Could you check a few things on this model? Use its own coordinates, in mm. Face numbers are marked on the shaded views. A direction names the side the tool comes from. Coordinates: 2 decimals unless noted, no trailing zeros. Loops run counter-clockwise (first coordinate to the right, second up) from the corner with the lowest first, then second, coordinate; pieces in that order, holes last. Notation, with made-up numbers: M 64,79.25 L 79,79.25 A13 ccw 79,88.25 Z; hole C 54.25,21.5 d10. An arc over 180 degrees is marked long. Write each question's results on one line, items separated by ' | '.
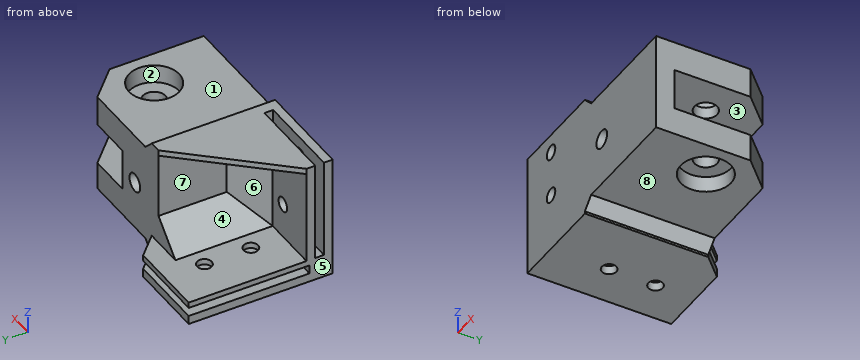
Autodesk Inventor part; units mm, degrees
ref_plane "Work Plane3" through (-127, -182.5, -3.81) normal (0, 0, -1) x (0, 1, 0)
ref_plane "YZ Plane" through (0, 0, 0) normal (1, 0, 0) x (0, 1, 0)
ref_plane "XZ Plane" through (0, 0, 0) normal (0, 1, 0) x (-1, 0, 0)
ref_plane "Work Plane1" through (0, 0, 0) normal (0, 0, 1) x (1, 0, 0)
ref_plane "Work Plane2" through (127, 182.5, 0) normal (1, 0, 0) x (0, 1, 0)
sketch "Sketch1" plane through (127, 182.5, 0) normal (1, 0, 0) x (0, 1, 0)
  line L0 (0, -3.81) -> (-365, -3.81)
  line L1 (0, 0) -> (0, -3.81)
  line L2 (0, 0) -> (-365, 0)
  line L3 (-365, 0) -> (-365, -3.81)
  line L4 (-371.35, 459.74) -> (-371.35, 2.54)
  line L5 (-367.54, 2.54) -> (-371.35, 2.54)
  line L6 (-367.54, 459.74) -> (-367.54, 2.54)
  line L7 (-367.54, 459.74) -> (-371.35, 459.74)
  line L8 (-367.54, 46.355) -> (-363.73, 46.355)
  line L9 (-321.185, -3.81) -> (-321.185, -7.62)
  line L10 (-321.185, -7.62) -> (-375.16, -7.62)
  line L11 (-375.16, -7.62) -> (-375.16, 46.355)
  line L12 (-363.73, 46.355) -> (-363.73, 2.54)
  line L13 (-363.73, 2.54) -> (-321.185, 2.54)
  line L14 (-321.185, 2.54) -> (-321.185, 0)
  line L15 (-321.185, 0) -> (-365, 0)
  line L16 (-365, 0) -> (-365, -3.81)
  line L17 (-365, -3.81) -> (-321.185, -3.81)
  line L18 (-371.35, 46.355) -> (-371.35, 41.275)
  line L19 (-371.35, 41.275) -> (-371.35, 2.54)
  line L20 (-371.35, 2.54) -> (-367.54, 2.54)
  line L21 (-367.54, 2.54) -> (-367.54, 46.355)
  line L22 (-375.16, 46.355) -> (-371.35, 46.355)
  line L23 (-367.54, 46.355) -> (-363.73, 46.355)
  point P0 (-182.5, 0)
  point P1 (-326.265, 0)
  point P2 (-326.265, -3.81)
  point P3 (-367.54, 41.275)
  dimension "d2" = 3.81
  dimension "d4" = 3.81
extrude "Extrusion1" add sketch "Sketch1" against normal blind 38.1 contours L9 L10 L11 L22 L4 L5 L6 L8 L12 L13 L14 L2 L3 L0
sketch "Sketch2" plane through (127, 182.5, 0) normal (1, 0, 0) x (0, 0, -1)
  line L0 (3.81, -365) -> (0, -365)
  line L1 (0, -365) -> (0, -321.185)
  line L2 (0, -321.185) -> (-2.54, -321.185)
  line L3 (-2.54, -321.185) -> (-2.54, -363.73)
  line L4 (-2.54, -363.73) -> (-46.355, -363.73)
  line L5 (-46.355, -363.73) -> (-46.355, -367.54)
  line L6 (-46.355, -367.54) -> (-2.54, -367.54)
  line L7 (-2.54, -367.54) -> (-2.54, -371.35)
  line L8 (-2.54, -371.35) -> (-46.355, -371.35)
  line L9 (-46.355, -371.35) -> (-46.355, -375.16)
  line L10 (-46.355, -375.16) -> (7.62, -375.16)
  line L11 (7.62, -375.16) -> (7.62, -321.185)
  line L12 (7.62, -321.185) -> (3.81, -321.185)
  line L13 (3.81, -321.185) -> (3.81, -365)
  line L14 (3.81, -321.185) -> (7.62, -321.185)
  line L15 (7.62, -375.16) -> (-46.355, -375.16)
  line L16 (7.62, -321.185) -> (-46.355, -321.185)
  line L17 (-46.355, -321.185) -> (-46.355, -375.16)
  line L18 (-46.355, -375.16) -> (7.62, -375.16)
  line L19 (7.62, -375.16) -> (7.62, -321.185)
  point P0 (0, -182.5)
extrude "Extrusion2" add sketch "Sketch2" along normal blind 5.08
sketch "Sketch3" plane through (88.9, -138.685, -3.81) normal (0, 1, 0) x (1, 0, 0)
  line L0 (38.1, -3.81) -> (0, -3.81)
  line L1 (0, -6.35) -> (0, -3.81)
  line L2 (38.1, -6.35) -> (0, -6.35)
  line L3 (38.1, -6.35) -> (38.1, -50.165)
  line L4 (38.1, -50.165) -> (43.18, -50.165)
  line L5 (43.18, 3.81) -> (43.18, -50.165)
  line L6 (0, 3.81) -> (43.18, 3.81)
  line L7 (0, 0) -> (0, 3.81)
  line L8 (38.1, 0) -> (0, 0)
  line L9 (38.1, 0) -> (38.1, -3.81)
  line L10 (43.18, -50.165) -> (43.18, 3.81)
  line L11 (43.18, -23.1775) -> (55.88, -23.1775)
  circle A0 centre (55.88, -23.1775) radius 4
  line L12 (55.88, -27.1775) -> (55.88, -32.2575)
  line L13 (55.88, -19.1775) -> (55.88, -14.0975)
  line L14 (59.88, -23.1775) -> (64.96, -23.1775)
  line L15 (43.18, -14.0975) -> (64.96, -14.0975)
  line L16 (64.96, -14.0975) -> (64.96, -32.2575)
  line L17 (64.96, -32.2575) -> (43.18, -32.2575)
  line L18 (43.18, -32.2575) -> (43.18, -14.0975)
  point P0 (-88.9, -3.81)
  dimension "d9" = 12.7
  dimension "d10" = 8
  dimension "d11" = 5.08
  dimension "d12" = 5.08
  dimension "d13" = 5.08
extrude "Extrusion3" add sketch "Sketch3" against normal up to surface (53.975 mm away) contours L15 L13 A0 L11 L5 | L5 L11 A0 L12 L17 | L15 L16 L14 A0 L13 | L12 A0 L14 L16 L17
sketch "Sketch4" plane through (132.08, -138.685, 28.4475) normal (0, 0, 1) x (1, 0, 0)
  line L0 (0, -53.975) -> (21.78, -53.975)
  line L1 (21.78, 0) -> (21.78, -53.975)
  line L2 (0, 0) -> (21.78, 0)
  line L3 (0, -53.975) -> (0, 0)
  line L4 (0, -53.975) -> (0, 0)
  line L5 (21.78, 0) -> (21.78, -53.975)
  line L6 (0, -45.966) -> (21.78, -45.966)
  line L7 (21.78, -45.966) -> (21.78, -26.916)
  line L8 (21.78, -26.916) -> (0, -26.916)
  line L9 (0, -26.916) -> (0, -45.966)
  line L10 (21.78, -45.966) -> (53.53, -45.966)
  line L11 (53.53, -45.966) -> (53.53, 0)
  line L12 (53.53, 0) -> (21.78, 0)
  line L13 (21.78, 0) -> (21.78, -45.966)
  circle A0 centre (37.655, -22.983) radius 11
  point P0 (-132.08, 138.685)
  dimension "d16" = 19.05
  dimension "d17" = 31.75
  dimension "d18" = 22
extrude "Extrusion4" add sketch "Sketch4" along normal blind 5.08 contours L3 L8 L1 L6 | L1 L12 L11 L10 | L3 L2 L1 L8
sketch "Sketch5" plane through (153.86, -138.685, 10.2875) normal (0, 0, -1) x (-1, 0, 0)
  circle A0 centre (-15.875, -22.983) radius 11
  line L0 (21.78, -45.966) -> (-31.75, -45.966)
  line L1 (-31.75, -45.966) -> (-31.75, 0)
  line L2 (-31.75, 0) -> (21.78, 0)
  line L3 (21.78, -45.966) -> (21.78, 0)
  point P0 (153.86, 138.685)
extrude "Extrusion5" add sketch "Sketch5" along normal blind 5.08
sketch "Sketch6" plane through (132.08, -138.685, 33.5275) normal (0, 0, 1) x (1, 0, 0)
  circle A0 centre (37.655, -22.983) radius 11
  line L0 (0, -45.966) -> (53.53, -45.966)
  line L1 (53.53, -45.966) -> (53.53, 0)
  line L2 (53.53, 0) -> (0, 0)
  line L3 (0, -45.966) -> (0, 0)
  point P0 (-132.08, 138.685)
extrude "Extrusion6" add sketch "Sketch6" along normal blind 8
sketch "Sketch7" plane through (132.08, -138.685, 28.4475) normal (0, 0, -1) x (-1, 0, 0)
  line L0 (-53.53, -45.966) -> (-53.53, 0)
  circle A0 centre (-37.655, -22.983) radius 11
  line L1 (0, -45.966) -> (-53.53, -45.966)
  line L2 (-53.53, -45.966) -> (-53.53, 0)
  line L3 (-53.53, 0) -> (0, 0)
  line L4 (0, -45.966) -> (0, 0)
  circle A1 centre (-37.655, -22.983) radius 5
  point P0 (132.08, 138.685)
  dimension "d25" = 10
extrude "Extrusion7" add sketch "Sketch7" against normal blind 5.08 contours A0
chamfer "Chamfer1" distance 4.7625 angle 45 1 edges at (132.08, -161.668, 41.5275)
sketch "Sketch8" plane through (153.86, -138.685, 10.2875) normal (0, 0, 1) x (1, 0, 0)
  circle A0 centre (15.875, -22.983) radius 5
  circle A1 centre (15.875, -22.983) radius 11
  point P0 (-153.86, 138.685)
extrude "Extrusion8" add sketch "Sketch8" against normal blind 5.08
sketch "Sketch9" plane through (153.86, -138.685, 5.2075) normal (0, 0, -1) x (-1, 0, 0)
  circle A0 centre (-15.875, -22.983) radius 5
  line L0 (-31.75, -45.966) -> (21.78, -45.966)
  line L1 (21.78, 0) -> (21.78, -45.966)
  line L2 (21.78, 0) -> (-31.75, 0)
  line L3 (-31.75, 0) -> (-31.75, -45.966)
  circle A1 centre (-15.875, -22.983) radius 11
  point P0 (153.86, 138.685)
extrude "Extrusion9" add sketch "Sketch9" along normal blind 7 contours L3 L2 L1 L0
chamfer "Chamfer2" distance 4.7625 angle 45 1 edges at (132.08, -161.668, -1.7925)
sketch "Sketch10" plane through (153.86, -184.651, 28.4475) normal (0, -1, 0) x (1, 0, 0)
  line L0 (4.875, -23.24) -> (26.875, -23.24)
  line L1 (-21.78, -18.16) -> (0, -18.16)
  line L2 (-21.78, -35.0025) -> (-21.78, -18.16)
  line L3 (-17.0175, -30.24) -> (-21.78, -35.0025)
  line L4 (31.75, -30.24) -> (-17.0175, -30.24)
  line L5 (31.75, -18.16) -> (31.75, -30.24)
  line L6 (0, -18.16) -> (31.75, -18.16)
  line L7 (4.875, 5.08) -> (26.875, 5.08)
  line L8 (0, 0) -> (-21.78, 0)
  line L9 (0, 0) -> (31.75, 0)
  line L10 (31.75, 0) -> (31.75, 13.08)
  line L11 (-17.0175, 13.08) -> (31.75, 13.08)
  line L12 (-21.78, 17.8425) -> (-17.0175, 13.08)
  line L13 (-21.78, 0) -> (-21.78, 17.8425)
  line L14 (0, 0) -> (31.75, 0)
  line L15 (31.75, -30.24) -> (0, -30.24)
  line L16 (0, -30.24) -> (0, 0)
  line L17 (0, 0) -> (31.75, 0)
  line L18 (31.75, 0) -> (31.75, -30.24)
  point P0 (-153.86, -28.4475)
extrude "Extrusion10" add sketch "Sketch10" along normal up to surface (8.009 mm away)
sketch "Sketch11" plane through (88.9, -185.04, 46.355) normal (0, 0, 1) x (1, 0, 0)
  line L0 (38.1, 3.81) -> (0, 3.81)
  line L1 (0, 0) -> (0, 3.81)
  line L2 (38.1, 0) -> (0, 0)
  line L3 (38.1, 0) -> (38.1, -3.81)
  line L4 (38.1, -3.81) -> (0, -3.81)
  line L5 (0, -7.62) -> (0, -3.81)
  line L6 (0, -7.62) -> (43.18, -7.62)
  line L7 (43.18, 46.355) -> (43.18, -7.62)
  line L8 (38.1, 46.355) -> (43.18, 46.355)
  line L9 (38.1, 46.355) -> (38.1, 3.81)
  line L10 (0, 0) -> (0, 3.81)
  line L11 (38.1, 46.355) -> (0, 3.81)
  line L12 (38.1, 3.81) -> (0, 3.81)
  line L13 (0, 3.81) -> (38.1, 3.81)
  line L14 (38.1, 3.81) -> (38.1, 46.355)
  point P0 (-88.9, 185.04)
extrude "Extrusion11" add sketch "Sketch11" against normal blind 2.54 contours L0 L11 L9
sketch "Sketch12" plane through (88.9, -181.23, 2.54) normal (0, 0, 1) x (1, 0, 0)
  circle A0 centre (17.78, 13.97) radius 3.175
  circle A1 centre (17.78, 34.29) radius 3.175
  circle A2 centre (17.78, 13.97) radius 3.175
  point P0 (-88.9, 181.23)
extrude "Extrusion12" cut sketch "Sketch12" against normal blind 45.4025
sketch "Sketch13" plane through (88.9, -181.23, 2.54) normal (0, 1, 0) x (1, 0, 0)
  circle A0 centre (17.78, -15.24) radius 3.175
  circle A1 centre (17.78, -35.56) radius 3.175
  point P0 (-88.9, 2.54)
extrude "Extrusion13" cut sketch "Sketch13" along normal mid plane 45.4025
chamfer "Chamfer3" distance 12.7 angle 45 2 edges at (127, -159.9575, 2.54) (127, -181.23, 23.1775)
chamfer "Chamfer4" distance 12.7 angle 45 2 edges at (185.61, -138.685, 4.2475) (185.61, -138.685, 34.9875)
sketch "Sketch14" plane through (88.9, -192.66, -7.62) normal (0, 0, -1) x (-1, 0, 0)
  circle A0 centre (-17.78, 25.4) radius 3.175
  circle A1 centre (-17.78, 45.72) radius 3.175
  line L0 (0, 0) -> (-43.18, 0)
  line L1 (0, 53.975) -> (0, 0)
  line L2 (0, 53.975) -> (-43.18, 53.975)
  line L3 (-43.18, 0) -> (-43.18, 53.975)
  line L4 (-43.18, 53.975) -> (-34.1997, 62.9553)
  line L5 (-43.18, 53.975) -> (-30.48, 53.975) construction
  line L6 (-34.1997, 62.9553) -> (0, 62.9553)
  line L7 (-25.4, 53.975) -> (0, 53.975)
  line L8 (0, 62.9553) -> (0, 53.975)
  line L9 (-47.9425, 53.975) -> (-43.18, 53.975)
  line L10 (-43.18, 53.975) -> (0, 53.975)
  point P0 (88.9, 192.66)
  dimension "d52" = 12.7
  dimension "d53" = 45
ref_plane "Work Plane3" through (-127, -182.5, -3.81) normal (0, 0, -1) x (0, 1, 0)
extrude "Extrusion14" add sketch "Sketch14" against normal up to surface (3.81 mm away) contours L2 L4 L6 L8
sketch "Sketch15" plane through (88.9, -182.5, 0) normal (0, 0, -1) x (-1, 0, 0)
  line L0 (-43.18, 43.815) -> (-34.1997, 52.7953)
  line L1 (-34.1997, 52.7953) -> (0, 52.7953)
  line L2 (-25.4, 43.815) -> (0, 43.815)
  line L3 (-38.1, 43.815) -> (-25.4, 43.815)
  line L4 (-38.1, 43.815) -> (-43.18, 43.815)
  line L5 (0, 0) -> (0, 52.7953)
  point P0 (88.9, 182.5)
extrude "Extrusion15" add sketch "Sketch15" against normal up to surface (2.54 mm away)
properties part number "Ystartnew"
(1) Which directions (+Z, -Z, +X, -X, +Y, -Y) give clear straight access to the entire face, cutting with the end or side of a thin tool? Please do the marked faces 1, 2, 3 and 4.
Reported:
face 1: +Z, +X, +Y, -Y | face 2: +Z | face 3: +X, +Y | face 4: -X, +Y
(2) Will these pins go through, and if not, where does the flat tip stop? P1, Ø5, axis at x = 106.68, z = 38.1, coming from the +Y side; P2, Ø12, axis at x = 139.5, y = -142, coming from the -Z side (3 decimals); P3, Ø3, axis at x = 138.5, y = -172, coming from the +Z side; P4, Ø20.5, axis at x = 97, z = 32.5, coming from the +Y side.
Reported:
P1: passes through | P2: stops at z = -5.135 | P3: stops at z = 41.53 | P4: stops at y = -181.23
(3) Please list where these lines run through material, in increasing order: probe 1 along Z at (x, y) = (100, -131.5); probe 2 along Y at (x, z) = (99, 4); probe 3 along Y at (x, z) = (125.5, 5) (3 decimals). Write a range as from..to.
Reported:
probe 1: z = -7.62..-3.81, 0..2.54 | probe 2: y = -192.66..-188.85, -185.04..-181.23 | probe 3: y = -192.66..-188.85, -185.04..-138.685
(4) Imagine slicing it at C-C, the plane y = -146.94. State how many separate pieces and enclosed holes the cut face has, and give its area (3 significant figures).
Reported:
separate pieces: 3 | enclosed holes: 1 | area: 2,180 mm2
(5) Imagine slicing it at A-A, the plane x = 144.78. List the corners of the cut face in (y, z) for me (1 decimal).
Reported:
outline: M -192.7,-1.8 L -138.7,-1.8 L -138.7,15.4 L -192.7,15.4 Z; M -192.7,23.4 L -138.7,23.4 L -138.7,41.5 L -192.7,41.5 Z
(6) Imagine slicing it at B-B, the plane z = 38.1. List the corners of the cut face in (x, y) for me (3 decimals).
Reported:
outline: M 88.9,-192.66 L 103.505,-192.66 L 103.505,-188.85 L 88.9,-188.85 Z; M 88.9,-185.04 L 103.505,-185.04 L 103.505,-181.23 L 88.9,-181.23 Z; M 109.855,-192.66 L 185.61,-192.66 L 185.61,-151.385 L 172.91,-138.685 L 127,-138.685 L 127,-168.53 L 114.3,-181.23 L 109.855,-181.23 L 109.855,-185.04 L 127,-185.04 L 127,-188.85 L 109.855,-188.85 Z; hole C 169.735,-161.668 d22
(7) If we mould it in two halves opening along Z, with no side actions, what happens to the marked faces 5, 6, 7 and 8? For each: released by +Z, released by -Z, zero draft, split by the parting line, or undercut.
Reported:
face 5: zero draft | face 6: undercut | face 7: undercut | face 8: released by -Z
